Autodesk Inventor part; units mm, degrees
ref_plane "YZ Plane" through (0, 0, 0) normal (1, 0, 0) x (0, 1, 0)
ref_plane "XZ Plane" through (0, 0, 0) normal (0, 1, 0) x (-1, 0, 0)
ref_plane "XY Plane" through (0, 0, 0) normal (0, 0, 1) x (1, 0, 0)
sketch "Sketch1" plane through (0, 0, 0) normal (1, 0, 0) x (0, 1, 0)
  line L0 (0, 0) -> (28, 0)
  line L1 (28, 0) -> (28, -2)
  line L2 (0, -2) -> (0, 0)
  line L3 (0, 0) -> (2, 0)
  line L4 (2, -28) -> (0, -28)
  line L5 (0, -28) -> (0, 0)
  line L6 (28, -2) -> (2, -2)
  line L7 (2, -2) -> (2, -28)
  dimension "d0" = 28
  dimension "d1" = 2
  dimension "d2" = 2
  dimension "d3" = 28
extrude "Extrusion1" add sketch "Sketch1" along normal blind 28
fillet "Fillet1" radius 2.5 5 edges at (28, 28, -1) (0, 28, -1) (28, 1, -28) (0, 1, -28) (14, 0, 0)
fillet "Fillet1" radius 8 1 edges at (14, 2, -2)
sketch "Sketch2" plane through (0, 2.5, 0) normal (0, 0, 1) x (1, 0, 0)
  circle A0 centre (14, 19.5) radius 1.85
  circle A1 centre (6, 11.5) radius 1.85
  circle A2 centre (22, 11.5) radius 1.85
  point P0 (0, -2.5)
extrude "Extrusion2" cut sketch "Sketch2" against normal through all
sketch "Sketch3" plane through (0, 0, -25.5) normal (0, -1, 0) x (1, 0, 0)
  circle A0 centre (6, 11.5) radius 1.85
  circle A1 centre (14, 3.5) radius 1.85
  circle A2 centre (22, 11.5) radius 1.85
  point P0 (0, 25.5)
extrude "Extrusion3" cut sketch "Sketch3" against normal through all
properties part number "sideplatemount"
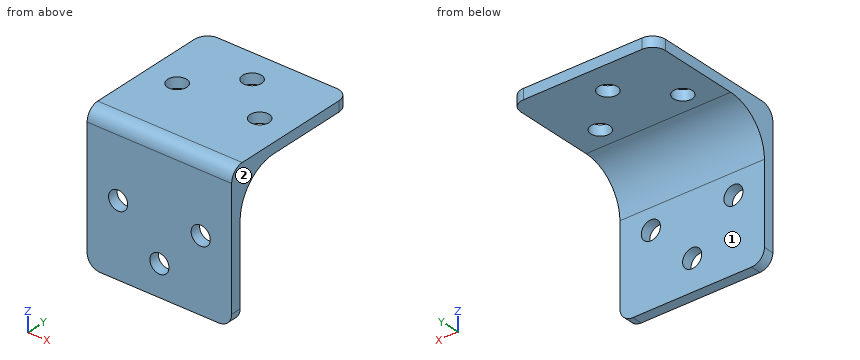
Input: part model. Units: mm. Frame: model coordinates. Face numbers are marked on the shaded views. A direction names the side the tool comes from. Coordinates: 2 decimals unless noted, no trailing zeros. Loops run counter-clockwise (first coordinate to the right, second up) from the corner with the lowest first, then second, coordinate; pieces in that order, holes last.
Q1. Contact query for flat-ended pins moving along their axis: pin 1 (8 mm diameter, centred on x = 20.5, y = 17, fed in from -Z); pin 2 (2 mm diameter, centred on x = 22, y = 14, fed in from -Z); pin 3 (6 mm diameter, centred on x = 22, z = -14, fed in from +Y); pin 4 (1 mm diameter, centred on x = 6.5, z = -4, fed in from +Y). Output: stop coordinate, or through.
Q2. Cut plane A-A (z = -14). Output: boundary loops of the cut face in (x, y).
Q3. Material intervals for line 1 (Z direction, x = 4.25, y = 20.75); line 2 (Y direction, x = 1, z = -15); line 3 (Z direction, x = 14, y = 0.9), sorted ascending.
Q4. Cut plane C-C (z = -22). Output: boundary loops of the cut face in (x, y).
Q5. Set-up query: the marked faces 1 and 2. Return all of +Z, -Z, +X, -X, +Y, -Y with unobstructed straight access to the full face (end or side cutting, diameter ignored); none if empty.
Q6. Cut plane D-D (y = 22). Output: boundary loops of the cut face in (x, z).
Q7. Cut plane B-B (y = 14). Output: boundary loops of the cut face in (x, z), then the cut area to 3 significant figures.
Working result:
1. pin 1: stops at z = -2
1. pin 2: passes through
1. pin 3: stops at y = 2
1. pin 4: stops at y = 5.34
2. outline: (0, 0) - (4.15, 0) - (4.15, 2) - (0, 2) - close; (7.85, 0) - (20.15, 0) - (20.15, 2) - (7.85, 2) - close; (23.85, 0) - (28, 0) - (28, 2) - (23.85, 2) - close
3. line 1: z = -2 to 0
3. line 2: y = 0 to 2
3. line 3: z = -28 to -23.85, -20.15 to -0.58
4. outline: (0, 0) - (12.15, 0) - (12.15, 2) - (0, 2) - close; (15.85, 0) - (28, 0) - (28, 2) - (15.85, 2) - close
5. face 1: -Z, +X, -X, +Y
5. face 2: +Z, -Z, +X, +Y, -Y
6. outline: (0, -2) - (12.15, -2) - (12.15, 0) - (0, 0) - close; (15.85, -2) - (28, -2) - (28, 0) - (15.85, 0) - close
7. outline: (0, -2) - (4.15, -2) - (4.15, 0) - (0, 0) - close; (7.85, -2) - (20.15, -2) - (20.15, 0) - (7.85, 0) - close; (23.85, -2) - (28, -2) - (28, 0) - (23.85, 0) - close
7. area: 41.2 mm2
